Verification items for the finished model (mm, model axes). A direction names the side the tool comes from. Coordinates: 2 decimals unless noted, no trailing zeros. Write each loop counter-clockwise with the first axis right and the second up, starting at its lowest first coordinate (ties: lowest second). Pieces come first, ordered by that corner, then holes. Notation, with made-up numbers: (-19.5, -25) -> (9.5, -25) arc R20 cw to (9.5, 6) -> close; hole circle Ø9 at (58, 12.5). An arc over 180 degrees is marked (long way). Answer in a Markdown table with one row per item.
```python
from build123d import *

# Parameters (mm, degrees)
F0_R      = 3.5
F0_R_2    = 1.5
F1_DEPTH  = 10
F1_FACE_R = 3.5
F2_DEPTH  = 5
F2_TAPER  = 22
F3_DEPTH  = 18
F4_R      = 1.3


with BuildPart() as f1:
    # F0 (on Top) → F1 (new body)
    with BuildSketch(Plane.XY):
        Circle(F0_R)
        Circle(F0_R_2, mode=Mode.SUBTRACT)
        Circle(F0_R_2)
    extrude(amount=F1_DEPTH)

    # F1_face (on face) → F2 (join)
    with BuildSketch(Plane.XY.offset(10)):
        Circle(F1_FACE_R)
    extrude(amount=F2_DEPTH, taper=F2_TAPER)

    # F0 (on Top) → F3 (join)
    with BuildSketch(Plane.XY):
        Circle(F0_R_2)
    extrude(amount=F3_DEPTH)

    # F4
    f4_edges = [f1.edges().sort_by_distance(p)[0] for p in [
        (-1.5, 0, 18),
    ]]
    fillet(f4_edges, radius=F4_R)


solid = f1.part
```
1. Section check A-A, the plane z = 8.25. Record the boundary of the cut face in (x, y).
Geometry says:
| item | result |
|---|---|
| outline | circle Ø7 at (0, 0) |
2. Depth check by flat-ended pin: P1, Ø3, axis at x = 2.5, z = 15, coming from the -Y side; P2, Ø2, axis at x = -0.5, z = 11.5, coming from the +Y side; P3, Ø3, axis at y = 2, z = 15, coming from the +X side. Enter the tip coordinate at first touch or a pass-through.
Geometry says:
| item | result |
|---|---|
| P1 | y = -1.32 |
| P2 | y = 3.28 |
| P3 | x = 1.66 |
3. Thickness scan on line 1 (Z direction, x = -0.25, y = 1); line 2 (Y direction, x = 2, z = 8.75); line 3 (X direction, y = -0.25, z = 6.75). Record the ranges inside material, lowest first. Write a range as from..to.
Geometry says:
| item | result |
|---|---|
| line 1 | 0..17.7 |
| line 2 | -2.87..2.87 |
| line 3 | -3.49..3.49 |
4. Tool access check on faces 1 (the cylindrical face through (3.233, -1.341, 4.93)), 2 (the cylindrical face through (-1.5, 0.07, 15.81)). Record the directions out of +Z, -Z, +X, -X, +Y, -Y that give a thin tool (end or side, any length) a straight path to the whole face; none if there is none.
Geometry says:
| item | result |
|---|---|
| face 1 | +Z, -Z |
| face 2 | +Z |
5. Section check B-B, the plane z = 13.25. Record the boundary of the cut face in (x, y), plus the area to 3 significant figures.
Geometry says:
| item | result |
|---|---|
| outline | circle Ø4.37 at (0, 0) |
| area | 15.0 mm^2 |
